Autodesk Inventor part; units mm, degrees
ref_plane "YZ Plane" through (0, 0, 0) normal (1, 0, 0) x (0, 1, 0)
ref_plane "XZ Plane" through (0, 0, 0) normal (0, 1, 0) x (-1, 0, 0)
ref_plane "XY Plane" through (0, 0, 0) normal (0, 0, 1) x (1, 0, 0)
sketch "Sketch1" plane through (0, 0, 0) normal (0, 0, 1) x (1, 0, 0)
  arc A0 (-24, 18.5) -> (-28, 14.5) centre (-24, 14.5) ccw
  line L0 (-28, 14.5) -> (-28, -14.5)
  arc A1 (-28, -14.5) -> (-24, -18.5) centre (-24, -14.5) ccw
  line L1 (-24, -18.5) -> (-22.5, -18.5)
  arc A2 (-18.5, -22.5) -> (-22.5, -18.5) centre (-22.5, -22.5) ccw
  line L2 (-18.5, -22.5) -> (-18.5, -24)
  arc A3 (-18.5, -24) -> (-14.5, -28) centre (-14.5, -24) ccw
  line L3 (-14.5, -28) -> (14.5, -28)
  arc A4 (14.5, -28) -> (18.5, -24) centre (14.5, -24) ccw
  line L4 (18.5, -24) -> (18.5, -22.5)
  arc A5 (22.5, -18.5) -> (18.5, -22.5) centre (22.5, -22.5) ccw
  line L5 (22.5, -18.5) -> (24, -18.5)
  arc A6 (24, -18.5) -> (28, -14.5) centre (24, -14.5) ccw
  line L6 (28, -14.5) -> (28, 14.5)
  arc A7 (28, 14.5) -> (24, 18.5) centre (24, 14.5) ccw
  line L7 (24, 18.5) -> (22.5, 18.5)
  arc A8 (18.5, 22.5) -> (22.5, 18.5) centre (22.5, 22.5) ccw
  line L8 (18.5, 22.5) -> (18.5, 24)
  arc A9 (18.5, 24) -> (14.5, 28) centre (14.5, 24) ccw
  line L9 (14.5, 28) -> (-14.5, 28)
  arc A10 (-14.5, 28) -> (-18.5, 24) centre (-14.5, 24) ccw
  line L10 (-18.5, 24) -> (-18.5, 22.5)
  arc A11 (-22.5, 18.5) -> (-18.5, 22.5) centre (-22.5, 22.5) ccw
  line L11 (-22.5, 18.5) -> (-24, 18.5)
  point P0 (0, 0)
  point P1 (0, 0)
extrude "Extrusion1" add sketch "Sketch1" along normal blind 33.5
properties part number "SERVO  KH56KM2U121 B"
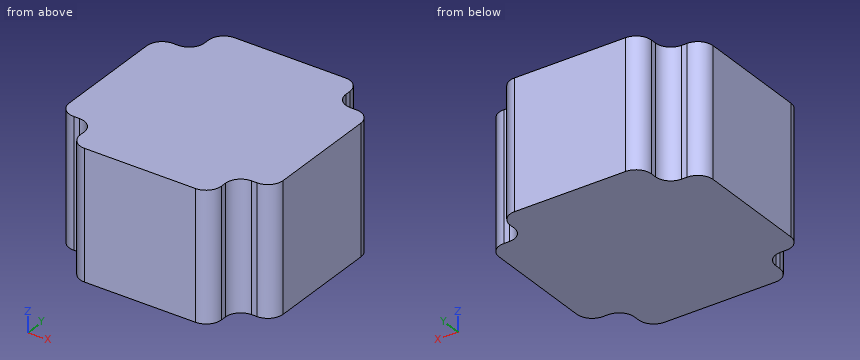
Here's how the part is built. I have some questions about the finished solid (model axes, mm). Coordinates: 2 decimals unless noted, no trailing zeros. Write each loop counter-clockwise with the first axis right and the second up, starting at its lowest first coordinate (ties: lowest second). Pieces come first, ordered by that corner, then holes. Notation, with made-up numbers: (39.25, 16.25) - (73.25, 16.25) arc R32 ccw to (73.25, 47.25) - close; hole circle Ø5 at (-18, 22.5). An arc over 180 degrees is marked (long way). One line per item, written item: value.
1) I need wall thicknesses on line 1 along X through (y, z) = (24, 8); line 2 along X through (y, z) = (16, 20). Which ranges of each line are inside material? Lowest first, please.
Model answer:
line 1: x = -18.5 to 18.5
line 2: x = -27.71 to 27.71
2) I'm going to push flat-ended pins straight in: P1, Ø1.6, axis at y = -23.5, z = 13.5, coming from the -X side; P2, Ø1.2, axis at y = 23.5, z = 13, coming from the +X side; P3, Ø1.2, axis at x = 23.5, z = 13.5, coming from the -Y side. Where does each tip first touch, or does it pass through?
Model answer:
P1: stops at x = -18.5
P2: stops at x = 18.5
P3: stops at y = -18.5
3) Suppose I cut it at B-B on x = 21. Write out the boundary of the cut face in (y, z), and give its area (3 significant figures).
Model answer:
outline: (-18.79, 0) - (18.79, 0) - (18.79, 33.5) - (-18.79, 33.5) - close
area: 1,260 mm²
4) Suppose I cut it at C-C on y = -25. Write out the boundary of the cut face in (x, z), and give its area (3 significant figures).
Model answer:
outline: (-18.37, 0) - (18.37, 0) - (18.37, 33.5) - (-18.37, 33.5) - close
area: 1,230 mm²
5) Suppose I cut it at A-A on z = 26. Write out the boundary of the cut face in (x, y), and give its area (3 significant figures).
Model answer:
outline: (-28, -14.5) arc R4 ccw to (-24, -18.5) - (-22.5, -18.5) arc R4 cw to (-18.5, -22.5) - (-18.5, -24) arc R4 ccw to (-14.5, -28) - (14.5, -28) arc R4 ccw to (18.5, -24) - (18.5, -22.5) arc R4 cw to (22.5, -18.5) - (24, -18.5) arc R4 ccw to (28, -14.5) - (28, 14.5) arc R4 ccw to (24, 18.5) - (22.5, 18.5) arc R4 cw to (18.5, 22.5) - (18.5, 24) arc R4 ccw to (14.5, 28) - (-14.5, 28) arc R4 ccw to (-18.5, 24) - (-18.5, 22.5) arc R4 cw to (-22.5, 18.5) - (-24, 18.5) arc R4 ccw to (-28, 14.5) - close
area: 2,760 mm²
